Here's the drawing with two shaded views (mm, measured from the low corner). I have some questions. A direction names the side the tool comes from. Give positions to 0.01 mm unless a question says otherwise; leave off trailing zeros. Loops run counter-clockwise (first coordinate to the right, second up) from the corner with the lowest first, then second, coordinate; pieces in that order, holes last. Notation, with made-up numbers: (41.5, 19) - (64.5, 19) arc R14 cw to (64.5, 26) - close; hole circle Ø3 at (73.25, 56). An arc over 180 degrees is marked (long way). Use a Markdown table: item, result. Add a question column.
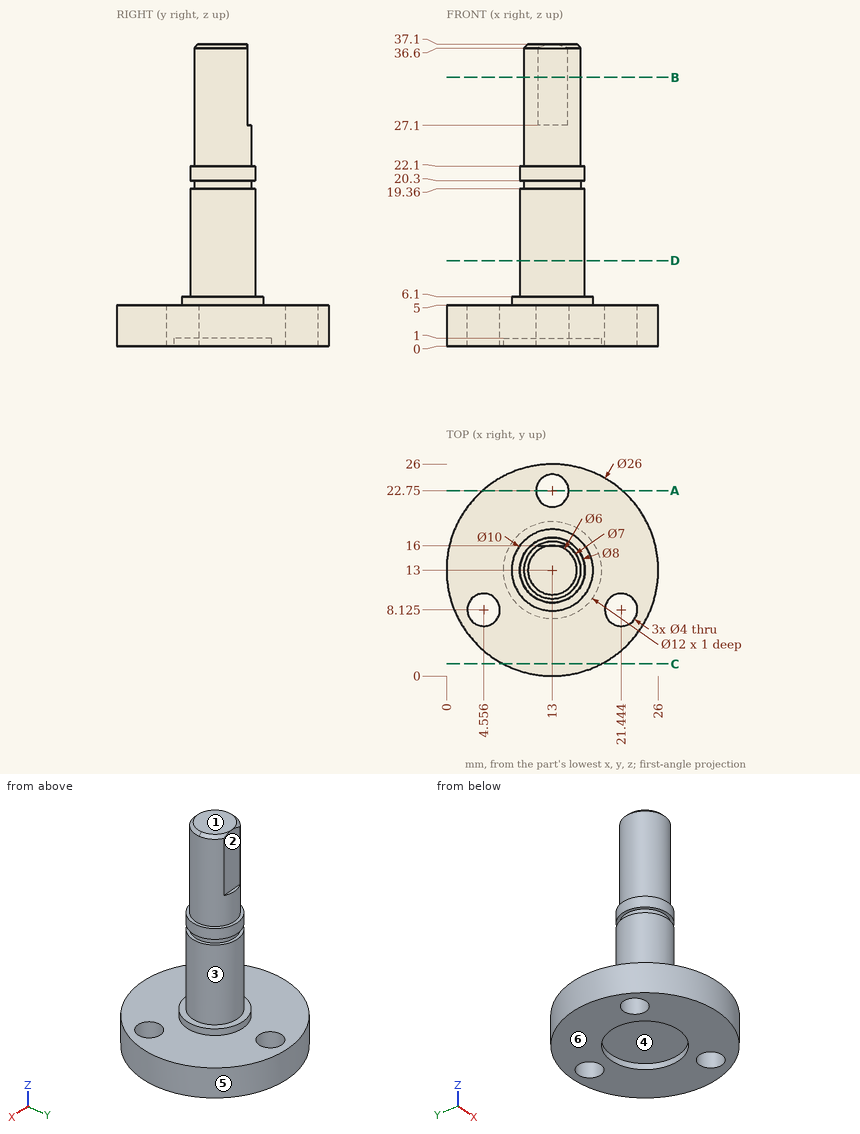
1. If we mould it in two halves opening along X, with no side actions, what happens to the marked faces 4, 5 and 6? For each: released by +X, released by -X, zero draft, split by the parting line, or undercut.
2. Please list where these lines run through material, in increasing order: line 1 along Y through (x, z) = (13, 0.6); line 2 along Z through (x, y) = (9.25, 13.5); line 3 along Z through (x, y) = (4.5, 21). Write a range as [from, to].
3. Suppose I cut it at B-B (z = 33). List the corners of the cut face in (x, y) for me, and give its area (3 significant figures).
4. Suppose I cut it at C-C (y = 1.5). List the corners of the cut face in (x, z) for me, and give its area (3 significant figures).
5. Suppose I cut it at A-A (y = 22.75). List the corners of the cut face in (x, z) for me.
6. Will these pins go through, and if not, where does the flat tip stop? P1, Ø6, axis at y = 9, z = 5, coming from the +X side; P2, Ø6.5, axis at x = 13, y = 22.75, coming from the +Z side; P3, Ø2, axis at y = 14.5, z = 24, coming from the -X side.
7. Suppose I cut it at D-D (z = 10.5). List the corners of the cut face in (x, y) for me.
8. On a 3-axis mill with a long thin cutter (end or side, diameter ignored), from which of +Z, -Z, +X, -X, +Y, -Y can I reach the whole of each face in a straight line? I mean the marked faces 1, 2 and 3. Say none if no direction works.
Results below:
| question | item | result |
|---|---|---|
| 1 | face 4 | undercut |
| 1 | face 5 | split by the parting line |
| 1 | face 6 | zero draft |
| 2 | line 1 | [0, 7], [19, 20.75], [24.75, 26] |
| 2 | line 2 | [1, 19.36], [20.3, 22.1] |
| 2 | line 3 | [0, 5] |
| 3 | outline | (11.2, 16) arc R3.5 ccw (long way) to (14.8, 16) - close |
| 3 | area | 37.3 mm² |
| 4 | outline | (6.94, 0) - (19.06, 0) - (19.06, 5) - (6.94, 5) - close |
| 4 | area | 60.6 mm² |
| 5 | outline | (4.4, 0) - (11, 0) - (11, 5) - (4.4, 5) - close; (15, 0) - (21.6, 0) - (21.6, 5) - (15, 5) - close |
| 6 | P1 | x = 25.96 |
| 6 | P2 | z = 5 |
| 6 | P3 | x = 9.54 |
| 7 | outline | circle Ø8 at (13, 13) |
| 8 | face 1 | +Z, +X, -X, +Y, -Y |
| 8 | face 2 | +Z, +X, -X, +Y |
| 8 | face 3 | +Z |
